Can you work these out from the model? Positions are in its coordinate system, mm. Face numbers are marked on the shaded views. A direction names the side the tool comes from. Coordinates: 2 decimals unless noted, no trailing zeros. Order: outer loops, then holes, each group sorted by start corner. A loop starts at its lowest first (then second) coordinate and runs counter-clockwise, first axis right, second up. Notation, with made-up numbers: M -33,-16.5 L 18,-16.5 A22 ccw 18,13.5 Z; hole C 86.5,-5.75 d6. An arc over 180 degrees is marked long. Answer as CSV lines item,"result". Start each with the question number.
1. I need wall thicknesses on line 1 along X through (y, z) = (-0.5, -5); line 2 along X through (y, z) = (-6.15, 12.75); line 3 along Z through (x, y) = (-19.7, -7.15). Which ranges of each line are inside material? Lowest first, please. Write a range as from..to.
2. If we section it at C-C (y = -3): List the corners of the cut face in (x, z) for me.
3. If we mould it in two halves opening along Z, with no side actions, what happens to the marked faces 6, 7 and 8? For each: released by +Z, released by -Z, zero draft, split by the parting line, or undercut.
4. Will these pins go through, and if not, where does the flat tip stop? pin 1 (0.6 mm diameter, centred on x = -13, z = 15, fed in from +Y); pin 2 (5 mm diameter, centred on x = -7, z = 5.5, fed in from +Y); pin 3 (5 mm diameter, centred on y = -4, z = 0, fed in from -X); pin 4 (3 mm diameter, centred on y = 5, z = 10.5, fed in from -X).
5. If we section it at A-A (x = 19.7): List the corners of the cut face in (y, z) for me, plus the area to 3 significant figures.
6. On a 3-axis mill with a long thin cutter (end or side, diameter ignored), from which of +Z, -Z, +X, -X, +Y, -Y can I reach the whole of each face in a straight line? I mean the marked faces 1, 2, 3, 4 and 5. Say none if no direction works.
7. If we section it at B-B (z = 12.75): List the corners of the cut face in (x, y) for me, plus the area to 3 significant figures.
8. If we section it at D-D (z = -4.5): List the corners of the cut face in (x, y) for me, plus the area to 3 significant figures.
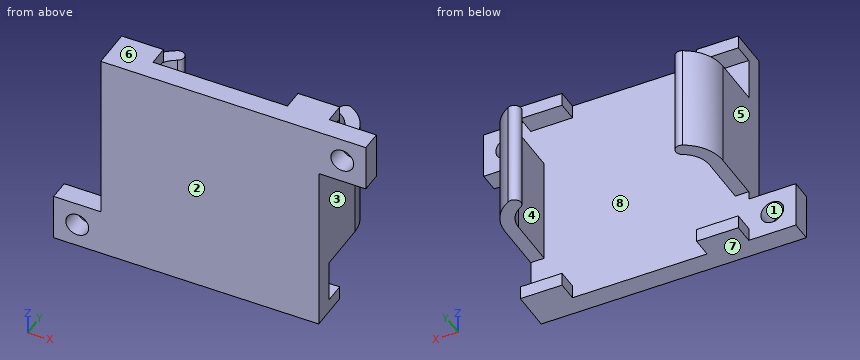
```python
from build123d import *

# Parameters (mm, degrees)
BOSS_EXTRUDE1_DEPTH      = 14.25
BOSS_EXTRUDE1_DEPTH_BACK = 14.25
BOSS_EXTRUDE2_START      = 14.25
SKETCH1_3_W              = 2
SKETCH1_3_H              = 3
SKETCH1_3_W_2            = 4.2
BOSS_EXTRUDE2_DEPTH      = 2
BOSS_EXTRUDE3_START      = -14.25
SKETCH1_6_W              = 2
SKETCH1_6_H              = 3
SKETCH1_6_W_2            = 4.2
BOSS_EXTRUDE3_DEPTH      = 2
BOSS_EXTRUDE4_DEPTH      = 8
BOSS_EXTRUDE4_DEPTH_BACK = 8
SKETCH1_7_W              = 2
SKETCH1_7_H              = 3
SKETCH1_7_R              = 1
BOSS_EXTRUDE5_START      = -8.2
SKETCH2_W                = 7
SKETCH2_H                = 7
SKETCH2_R                = 1.7
BOSS_EXTRUDE5_DEPTH      = 3


with BuildPart() as part:
    # Sketch1 → Boss-Extrude1 (new, two sides: drawn at the far end of the back side and taken through both)
    with BuildSketch(Plane.XY.offset(-BOSS_EXTRUDE1_DEPTH_BACK)):
        Polygon((-14.2, -5.2), (-16.2, -5.2), (-16.2, -8.2), (16.2, -8.2), (16.2, -5.2), (14.2, -5.2), (10, -5.2), (-10, -5.2), align=None)
    extrude(amount=BOSS_EXTRUDE1_DEPTH + BOSS_EXTRUDE1_DEPTH_BACK)

    # Sketch1<3> → Boss-Extrude2 (add)
    with BuildSketch(Plane.XY.offset(BOSS_EXTRUDE2_START)):
        Polygon((-14.2, -5.2), (-16.2, -5.2), (-16.2, -8.2), (16.2, -8.2), (16.2, -5.2), (14.2, -5.2), (10, -5.2), (-10, -5.2), align=None)
        with Locations((-15.2, -3.7)):
            Rectangle(SKETCH1_3_W, SKETCH1_3_H)
        with Locations((-12.1, -3.7)):
            Rectangle(SKETCH1_3_W_2, SKETCH1_3_H)
        with Locations((12.1, -3.7)):
            Rectangle(SKETCH1_3_W_2, SKETCH1_3_H)
        with Locations((15.2, -3.7)):
            Rectangle(SKETCH1_3_W, SKETCH1_3_H)
    extrude(amount=BOSS_EXTRUDE2_DEPTH)

    # Sketch1<6> → Boss-Extrude3 (add)
    with BuildSketch(Plane.XY.offset(BOSS_EXTRUDE3_START)):
        with Locations((-15.2, -3.7)):
            Rectangle(SKETCH1_6_W, SKETCH1_6_H)
        with Locations((-12.1, -3.7)):
            Rectangle(SKETCH1_6_W_2, SKETCH1_6_H)
        Polygon((-14.2, -5.2), (-16.2, -5.2), (-16.2, -8.2), (16.2, -8.2), (16.2, -5.2), (14.2, -5.2), (10, -5.2), (-10, -5.2), align=None)
        with Locations((12.1, -3.7)):
            Rectangle(SKETCH1_6_W_2, SKETCH1_6_H)
        with Locations((15.2, -3.7)):
            Rectangle(SKETCH1_6_W, SKETCH1_6_H)
    extrude(amount=-BOSS_EXTRUDE3_DEPTH)

    # Sketch1<7> → Boss-Extrude4 (add, two sides: drawn at the far end of the back side and taken through both)
    with BuildSketch(Plane.XY.offset(-BOSS_EXTRUDE4_DEPTH_BACK)):
        with Locations((-15.2, -3.7)):
            Rectangle(SKETCH1_7_W, SKETCH1_7_H)
        with BuildLine():
            Line((-16.2, 2.2), (-16.2, -2.2))
            Line((-16.2, -2.2), (-14.2, -2.2))
            Line((-14.2, -2.2), (-14.2, 2.2))
            ThreePointArc((-14.2, 2.2), (-13.617601514, 4.278460942), (-12.040000055, 5.751675632))
            ThreePointArc((-12.040000055, 5.751675632), (-13.387918942, 6.179594627), (-12.959999953, 7.527513516))
            ThreePointArc((-12.959999953, 7.527513516), (-15.326402233, 5.317691476), (-16.2, 2.2))
        make_face()
        with Locations((-12.5, 6.639594576)):
            Circle(SKETCH1_7_R)
        with Locations((12.5, 6.639594576)):
            Circle(SKETCH1_7_R)
        with BuildLine():
            Line((14.2, 2.2), (14.2, -2.2))
            Line((14.2, -2.2), (16.2, -2.2))
            Line((16.2, -2.2), (16.2, 2.2))
            ThreePointArc((16.2, 2.2), (15.326402246, 5.317691455), (12.959999996, 7.527513493))
            ThreePointArc((12.959999996, 7.527513493), (13.354400373, 7.15920982), (13.5, 6.639594576))
            ThreePointArc((13.5, 6.639594576), (13.019615242, 5.785194201), (12.039999999, 5.751675662))
            ThreePointArc((12.039999999, 5.751675662), (13.617601498, 4.27846097), (14.2, 2.2))
        make_face()
        with Locations((15.2, -3.7)):
            Rectangle(SKETCH1_7_W, SKETCH1_7_H)
    extrude(amount=BOSS_EXTRUDE4_DEPTH + BOSS_EXTRUDE4_DEPTH_BACK)

    # Sketch2 → Boss-Extrude5 (add)
    # profile 1 of 2: a face of its own
    with BuildSketch(Plane(origin=(0, 0, 0), x_dir=(1, 0, 0), z_dir=(0, 1, 0)).offset(BOSS_EXTRUDE5_START)):
        with Locations((-19.7, 12.75)):
            Rectangle(SKETCH2_W, SKETCH2_H)
        with Locations(Location((-19.7, 12.75, 0), (0, 0, 90))):
            Circle(SKETCH2_R, mode=Mode.SUBTRACT)
    # profile 2 of 2: a face of its own
    with BuildSketch(Plane(origin=(0, 0, 0), x_dir=(1, 0, 0), z_dir=(0, 1, 0)).offset(BOSS_EXTRUDE5_START)):
        with Locations((19.7, -12.75)):
            Rectangle(SKETCH2_W, SKETCH2_H)
        with Locations(Location((19.7, -12.75, 0), (0, 0, 90))):
            Circle(SKETCH2_R, mode=Mode.SUBTRACT)
    extrude(amount=BOSS_EXTRUDE5_DEPTH)


solid = part.part
```
Solved:
1,line 1,"-16.2..-14.2, 14.2..16.2"
1,line 2,"-16.2..18, 21.4..23.2"
1,line 3,"-16.25..-14.45, -11.05..-9.25"
2,outline,"M -16.2,-16.25 L -10,-16.25 L -10,-14.25 L -16.2,-14.25 Z; M -16.2,-8 L -14.2,-8 L -14.2,8 L -16.2,8 Z; M -16.2,14.25 L -10,14.25 L -10,16.25 L -16.2,16.25 Z; M 10,-16.25 L 16.2,-16.25 L 16.2,-14.25 L 10,-14.25 Z; M 10,14.25 L 16.2,14.25 L 16.2,16.25 L 10,16.25 Z; M 14.2,-8 L 16.2,-8 L 16.2,8 L 14.2,8 Z"
3,face 6,"released by +Z"
3,face 7,"released by -Z"
3,face 8,"undercut"
4,pin 1,"y = -2.2"
4,pin 2,"y = -5.2"
4,pin 3,"x = -16.2"
4,pin 4,"through"
5,outline,"M -8.2,9.25 L -5.2,9.25 L -5.2,11.05 L -8.2,11.05 Z; M -8.2,14.45 L -5.2,14.45 L -5.2,16.25 L -8.2,16.25 Z"
5,area,"10.8 mm²"
6,face 1,"+Y, -Y"
6,face 2,"+Z, -Z, +X, -X, -Y"
6,face 3,"-Z, +X, +Y, -Y"
6,face 4,"none"
6,face 5,"+Z, -X, +Y, -Y"
7,outline,"M -16.2,-8.2 L 18,-8.2 L 18,-5.2 L -16.2,-5.2 Z; M 21.4,-8.2 L 23.2,-8.2 L 23.2,-5.2 L 21.4,-5.2 Z"
7,area,"108 mm²"
8,outline,"M -16.2,-8.2 L 16.2,-8.2 L 16.2,2.2 A6 ccw 12.96,7.53 A1 ccw 12.04,5.75 A4 cw 14.2,2.2 L 14.2,-5.2 L -14.2,-5.2 L -14.2,2.2 A4 cw -12.04,5.75 A1 ccw -12.96,7.53 A6 ccw -16.2,2.2 Z"
8,area,"152 mm²"
